Geometry: see drawing. Coordinates: mm, zero at the bounding-box minimum. A direction names the side the tool comes from. Coordinates: 2 decimals unless noted, no trailing zeros. Order: outer loops, then holes, each group sorted by start corner. A loop starts at its lowest first (then second) coordinate and runs counter-clockwise, first axis right, second up.
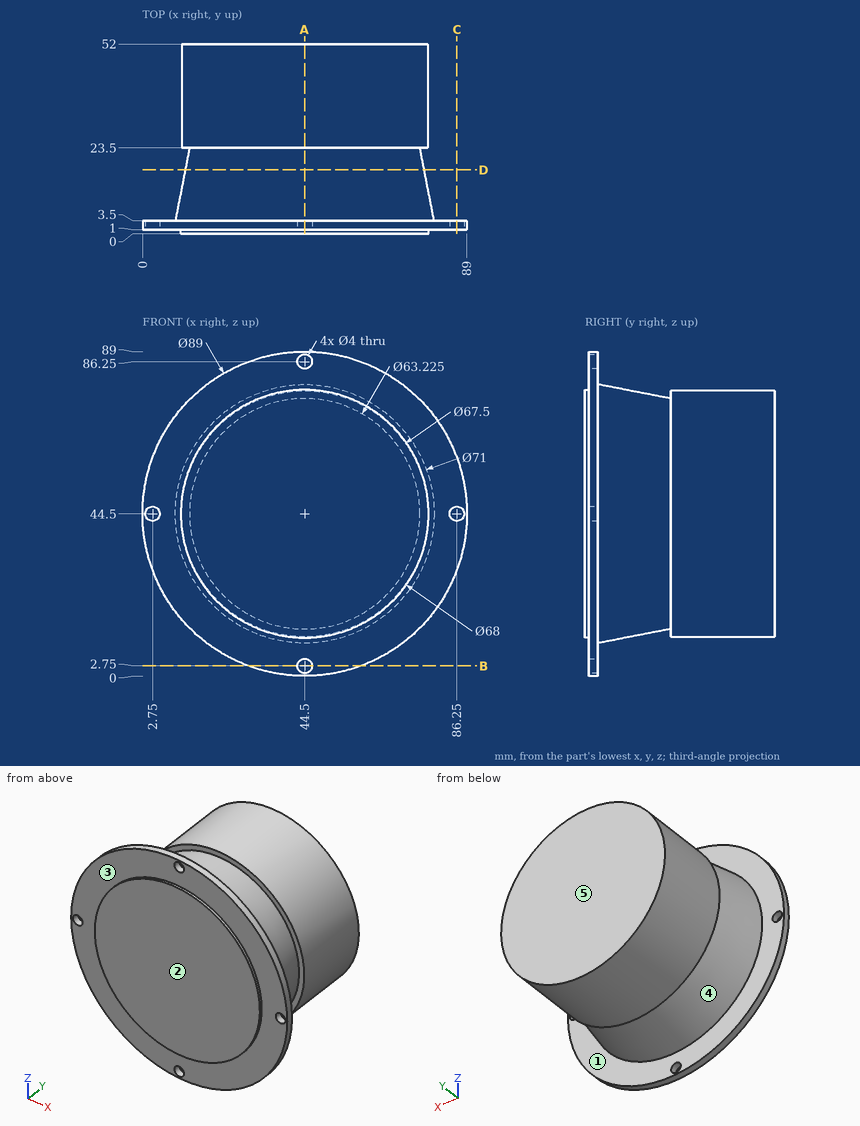
Q1. Material intervals for line 1 along X through (y, z) = (1.95, 44.5); line 2 along Y through (x, z) = (10, 26.5); line 3 along Z through (x, y) = (44, 2), sorted ascending.
Solutions:
line 1: x = 0 to 0.75, 4.75 to 84.25, 88.25 to 89
line 2: y = 1 to 3.5
line 3: z = 0 to 0.81, 4.69 to 84.31, 88.19 to 89
Q2. Set-up query: the marked faces 1 and 2. Return all of +Z, -Z, +X, -X, +Y, -Y with unobstructed straight access to the full face (end or side cutting, diameter ignored); none if empty.
Solutions:
face 1: +Y
face 2: +Z, -Z, +X, -X, -Y
Q3. Section query B-B on z = 2.75. Output: boundary loops of the cut face in (x, y).
Solutions:
outline: (29.1, 1) - (42.5, 1) - (42.5, 3.5) - (29.1, 3.5) - close; (46.5, 1) - (59.9, 1) - (59.9, 3.5) - (46.5, 3.5) - close
Q4. Section query A-A on x = 44.5. Output: boundary loops of the cut face in (y, z).
Solutions:
outline: (0, 10.5) - (1, 10.5) - (1, 4.75) - (3.5, 4.75) - (3.5, 9) - (23.5, 12.89) - (23.5, 10.75) - (52, 10.75) - (52, 78.25) - (23.5, 78.25) - (23.5, 76.11) - (3.5, 80) - (3.5, 84.25) - (1, 84.25) - (1, 78.5) - (0, 78.5) - close; (1, 0) - (3.5, 0) - (3.5, 0.75) - (1, 0.75) - close; (1, 88.25) - (3.5, 88.25) - (3.5, 89) - (1, 89) - close
Q5. Section query C-C on x = 86.25. Output: boundary loops of the cut face in (y, z), plus the area to 3 significant figures.
Solutions:
outline: (1, 29.1) - (3.5, 29.1) - (3.5, 42.5) - (1, 42.5) - close; (1, 46.5) - (3.5, 46.5) - (3.5, 59.9) - (1, 59.9) - close
area: 67.0 mm2
Q6. Pull-direction query (Y, two-part tool) for the marked faces 3, 4 and 5; classes: pulls with the +Y half, pulls with the -Y half, needs draft (parallel to the pull), parting line crosses it, or undercut.
Solutions:
face 3: pulls with the -Y half
face 4: undercut
face 5: pulls with the +Y half
Q7. Pin query (flat end, axial travel): P1, Ø10, axis at x = 77.5, y = 19.5, coming from the -Z side (1 decimal); P2, Ø3.5, axis at x = 44.5, z = 2.75, coming from the +Y side; P3, Ø6.5, axis at x = 2.75, z = 44.5, coming from the +Y side; P4, Ø8, axis at x = 25, y = 14, coming from the -Z side. Return the tip coordinate at first contact, or that it passes through.
Solutions:
P1: stops at z = 28
P2: passes through
P3: stops at y = 3.5
P4: stops at z = 14.67
Q8. Section query D-D on y = 17.5. Output: boundary loops of the cut face in (x, z), plus the area to 3 significant figures.
Solutions:
outline: circle Ø65.56 at (44.5, 44.5)
area: 3,380 mm2
